from build123d import *

# Parameters (mm, degrees)
SKETCH1_R           = 5.5
SKETCH1_W           = 20
SKETCH1_H           = 3
BOSS_EXTRUDE2_DEPTH = 3


with BuildPart() as part:
    # Sketch1 → Boss-Extrude2 (new body)
    with BuildSketch(Plane(origin=(0, 0, 0), x_dir=(0, 0, -1), z_dir=(1, 0, 0))):
        Polygon((0, 0), (50, 0), (50, 11), (53, 11), (53, 31), (50, 31), (50, 53), (53, 53), (53, 73), (50, 73), (50, 84), (0, 84), (0, 73), (-3, 73), (-3, 53), (0, 53), (0, 31), (-3, 31), (-3, 11), (0, 11), align=None)
        with Locations((25, 16.2)):
            Circle(SKETCH1_R, mode=Mode.SUBTRACT)
        with Locations((25, 3.5)):
            Rectangle(SKETCH1_W, SKETCH1_H, mode=Mode.SUBTRACT)
    extrude(amount=BOSS_EXTRUDE2_DEPTH)


solid = part.part
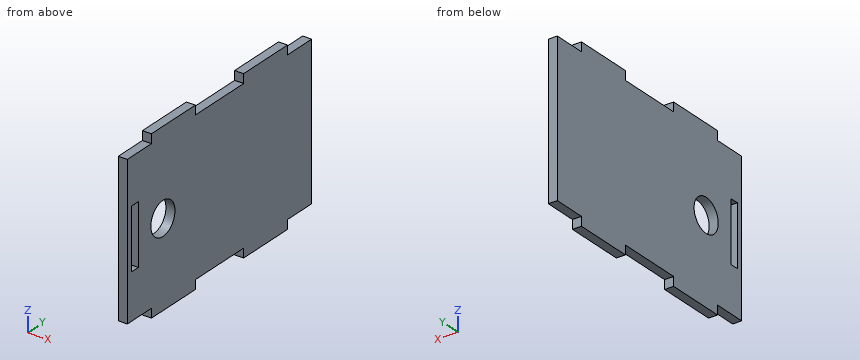
Can you work these out from the model? Positions are in its coordinate system, mm. Coordinates: 2 decimals unless noted, no trailing zeros. Order: outer loops, then holes, each group sorted by start corner. A loop starts at its lowest first (then second) coordinate and runs counter-clockwise, first axis right, second up. Notation, with made-up numbers: (0, -38.75) - (52, -38.75) arc R17 ccw to (52, -8.75) - close; hole circle Ø10 at (29, 80). An arc over 180 degrees is marked (long way). Answer as a JSON object with one key per item and string values. Group by question number.
Q1. Imagine slicing it at C-C (x = 1.75). Please give me the cut outline in (y, z).
Q2. Imagine slicing it at A-A (y = 16.2). Please give me the cut outline in (x, z).
Q3. Will these pins go through, and if not, where does the flat tip stop? P1, Ø0.9, axis at x = 1, y = 78, coming from the -Z side; P2, Ø14.5, axis at y = 16.2, z = -25, coming from the -X side; P3, Ø1.5, axis at x = 1.5, z = 1.5, coming from the +Y side; P4, Ø0.9, axis at x = 2, z = 1.5, coming from the -Y side.
Q4. Imagine slicing it at B-B (z = -25). Please give me the cut outline in (x, y).
Q5. Imagine slicing it at D-D (y = 40). Please give me the cut outline in (x, z), and give its area (3 significant figures).
Q6. I need wall thicknesses on line 1 (Y direction, x = 2.4, z = -25); line 2 (Y direction, x = 0.35, z = 0.5); line 3 (Y direction, x = 0.35, z = -22.5). Which ranges of each line are inside material? Lowest first, please. Write a range as from..to.
Determined:
{
 "1": {"outline": "(0, -50) - (11, -50) - (11, -53) - (31, -53) - (31, -50) - (53, -50) - (53, -53) - (73, -53) - (73, -50) - (84, -50) - (84, 0) - (73, 0) - (73, 3) - (53, 3) - (53, 0) - (31, 0) - (31, 3) - (11, 3) - (11, 0) - (0, 0) - close; hole (2, -35) - (5, -35) - (5, -15) - (2, -15) - close; hole circle Ø11 at (16.2, -25)"},
 "2": {"outline": "(0, -53) - (3, -53) - (3, -30.5) - (0, -30.5) - close; (0, -19.5) - (3, -19.5) - (3, 3) - (0, 3) - close"},
 "3": {"P1": "stops at z = -50", "P2": "stops at x = 0", "P3": "stops at y = 73", "P4": "stops at y = 11"},
 "4": {"outline": "(0, 0) - (3, 0) - (3, 2) - (0, 2) - close; (0, 5) - (3, 5) - (3, 10.7) - (0, 10.7) - close; (0, 21.7) - (3, 21.7) - (3, 84) - (0, 84) - close"},
 "5": {"outline": "(0, -50) - (3, -50) - (3, 0) - (0, 0) - close", "area": "150 mm2"},
 "6": {"line 1": "y = 0..2, 5..10.7, 21.7..84", "line 2": "y = 11..31, 53..73", "line 3": "y = 0..2, 5..11.3, 21.1..84"}
}
